```python
from build123d import *

# Parameters (mm, degrees)
ESQUISSE1_W             = 57
ESQUISSE1_H             = 114
BOSS_EXTRU_1_DEPTH      = 1.5
ESQUISSE3_R             = 1.75
ESQUISSE3_W             = 57
ESQUISSE3_H             = 106.5
ESQUISSE3_W_2           = 53
ESQUISSE3_H_2           = 102.5
BOSS_EXTRU_2_DEPTH      = 5
ENL_V_START             = -12
ESQUISSE4_R             = 1.75
ENL_V_MAT_EXTRU_1_DEPTH = 12


with BuildPart() as part:
    # Esquisse1 → Boss.-Extru.1 (new body)
    with BuildSketch(Plane.XY):
        with Locations((28.5, 57)):
            Rectangle(ESQUISSE1_W, ESQUISSE1_H)
    extrude(amount=BOSS_EXTRU_1_DEPTH)

    # Esquisse3 → Boss.-Extru.2 (add)
    # profile 1 of 3: a face of its own
    with BuildSketch(Plane(origin=(0, 0, 0), x_dir=(-1, 0, 0), z_dir=(0, 0, -1))):
        with Locations((-4, 4)):
            Circle(ESQUISSE3_R)
    # profile 2 of 3: a face of its own
    with BuildSketch(Plane(origin=(0, 0, 0), x_dir=(-1, 0, 0), z_dir=(0, 0, -1))):
        with Locations((-53, 4)):
            Circle(ESQUISSE3_R)
    # profile 3 of 3: a face of its own
    with BuildSketch(Plane(origin=(0, 0, 0), x_dir=(-1, 0, 0), z_dir=(0, 0, -1))):
        with Locations((-28.5, 60.75)):
            Rectangle(ESQUISSE3_W, ESQUISSE3_H)
        with Locations((-28.5, 60.75)):
            Rectangle(ESQUISSE3_W_2, ESQUISSE3_H_2, mode=Mode.SUBTRACT)
    extrude(amount=BOSS_EXTRU_2_DEPTH)

    # Esquisse4 → Enlèv. mat.-Extru.1 (cut)
    with BuildSketch(Plane(origin=(0, 0, -5), x_dir=(-1, 0, 0), z_dir=(0, 0, -1)).offset(ENL_V_START)):
        with Locations((-4, 4)):
            Circle(ESQUISSE4_R)
        with Locations((-53, 4)):
            Circle(ESQUISSE4_R)
    extrude(amount=ENL_V_MAT_EXTRU_1_DEPTH, mode=Mode.SUBTRACT)


solid = part.part
```
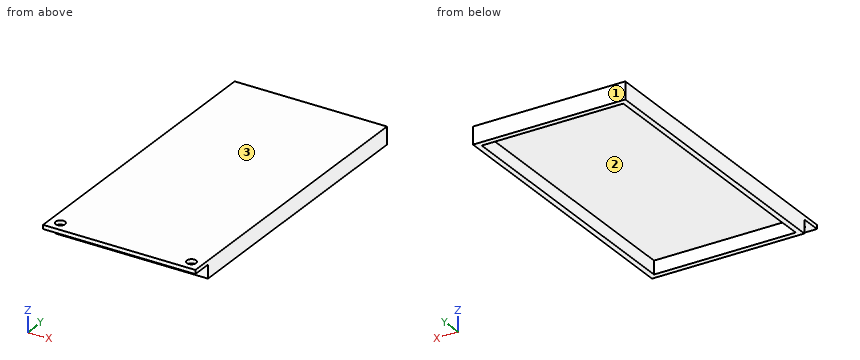
Geometry: final body of the model. Coordinates: model frame, mm. Face numbers are marked on the shaded views. Give positions to 0.01 mm unless a question says otherwise; leave off trailing zeros. Order: outer loops, then holes, each group sorted by start corner. A loop starts at its lowest first (then second) coordinate and runs counter-clockwise, first axis right, second up. Notation, with made-up numbers: (42, 56.25) -> (79, 56.25) arc R33 cw to (79, 86.25) -> close; hole circle Ø10 at (41, 26.25). An arc over 180 degrees is marked (long way). Write each question's results on one line, items separated by ' | '. Start each with the question number.
1) Section D-D (x = 17). Return loops of the section in (y, z).
2) Section C-C (y = 46). Return loops of the section in (x, z).
3) Line query: line 1 (X direction, y = 4, z = 0.3); line 2 (Y direction, x = 4, z = 1.1); line 3 (X direction, y = 74.5, z = -2.25). Output: solid intervals per line, ascending. Write a range as from..to.
4) Section B-B (x = 53). Return loops of the section in (y, z).
5) First-contact query: pin 1 (2.5 mm diameter, centred on y = 82, z = -3.5, fed in from -X); pin 2 (4 mm diameter, centred on x = 53, y = 4, fed in from -Z); pin 3 (2.5 mm diameter, centred on x = 27, z = -2.5, fed in from -Y). Flat tips, straight axial feed; report the tip coordinate or a pass-through.
6) Draft query along Y for the marked faces 1, 2 and 3. Return one class per face: pulls with the +Y half, pulls with the -Y half, needs draft (parallel to the pull), parting line crosses it, or undercut.
7) Section A-A (z = -1.75). Return loops of the section in (x, y), then the cut area to 3 significant figures.
Calculated:
1) outline: (0, 0) -> (7.5, 0) -> (7.5, -5) -> (9.5, -5) -> (9.5, 0) -> (112, 0) -> (112, -5) -> (114, -5) -> (114, 1.5) -> (0, 1.5) -> close
2) outline: (0, -5) -> (2, -5) -> (2, 0) -> (55, 0) -> (55, -5) -> (57, -5) -> (57, 1.5) -> (0, 1.5) -> close
3) line 1: 0..2.25, 5.75..51.25, 54.75..57 | line 2: 0..2.25, 5.75..114 | line 3: 0..2, 55..57
4) outline: (0, 0) -> (2.25, 0) -> (2.25, 1.5) -> (0, 1.5) -> close; (5.75, 0) -> (7.5, 0) -> (7.5, -5) -> (9.5, -5) -> (9.5, 0) -> (112, 0) -> (112, -5) -> (114, -5) -> (114, 1.5) -> (5.75, 1.5) -> close
5) pin 1: x = 0 | pin 2: z = 0 | pin 3: y = 7.5
6) face 1: pulls with the +Y half | face 2: undercut | face 3: needs draft
7) outline: (0, 7.5) -> (57, 7.5) -> (57, 114) -> (0, 114) -> close; hole (2, 9.5) -> (55, 9.5) -> (55, 112) -> (2, 112) -> close | area: 638 mm2
